```python
from build123d import *

# Parameters (mm, degrees)
SKETCH1_R           = 3.4
SKETCH1_R_2         = 2.45
BOSS_EXTRUDE1_DEPTH = 5.5
BOSS_EXTRUDE2_START = -1.5
SKETCH2_R           = 8.4
SKETCH2_R_2         = 3.4
BOSS_EXTRUDE2_DEPTH = 1.5
FILLET1_R           = 2
FILLET2_R           = 2


with BuildPart() as part:
    # Sketch1 → Boss-Extrude1 (new body)
    with BuildSketch(Plane.XY):
        Circle(SKETCH1_R)
        Circle(SKETCH1_R_2, mode=Mode.SUBTRACT)
    extrude(amount=BOSS_EXTRUDE1_DEPTH)

    # Sketch2 → Boss-Extrude2 (add)
    with BuildSketch(Plane.XY.offset(5.5).offset(BOSS_EXTRUDE2_START)):
        Circle(SKETCH2_R)
        Circle(SKETCH2_R_2, mode=Mode.SUBTRACT)
    extrude(amount=BOSS_EXTRUDE2_DEPTH)

    # Fillet1
    fillet1_edges = [part.edges().sort_by_distance(p)[0] for p in [
        (-3.4, 0, 4),
    ]]
    fillet(fillet1_edges, radius=FILLET1_R)

    # Fillet2
    fillet2_edges = [part.edges().sort_by_distance(p)[0] for p in [
        (-2.45, 0, 5.5),
    ]]
    fillet(fillet2_edges, radius=FILLET2_R)


solid = part.part
```
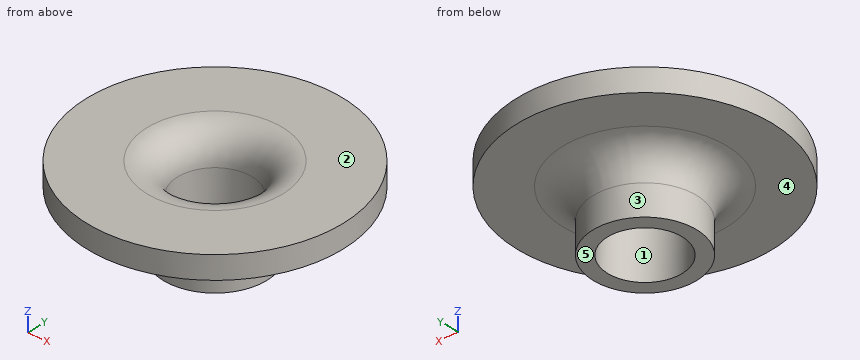
Part model, mm, in its own coordinate system. Face numbers are marked on the shaded views. A direction names the side the tool comes from. Coordinates: 2 decimals unless noted, no trailing zeros. Loops run counter-clockwise (first coordinate to the right, second up) from the corner with the lowest first, then second, coordinate; pieces in that order, holes last. Notation, with made-up numbers: (-39, -0.75) - (-31, -0.75) arc R16 ccw to (-31, 27.25) - close; hole circle Ø4 at (59, -27). An arc over 180 degrees is marked (long way). Write item = value, one per line. Start each with the question number.
Item 1: Cut at A-A, the plane y = 0. Give the cut face in (x, z).
Item 2: 3-axis set-ups, long thin cutter, end or side, ignore diameter. For the marked faces 4 and 5: which of +Z, -Z, +X, -X, +Y, -Y reach the whole face in a straight line?
Item 3: Flat gauge pins, fed straight in: pin 1 Ø2 at (y, z) = (5.5, 4.5) entering from -X; pin 2 Ø1.5 at (y, z) = (6.5, 2) entering from -X; pin 3 Ø1.5 at (x, y) = (3.5, 6.5) entering from -Z. Where does each tip first touch, or does it go through?
Item 4: Mould opens along X. For the marked faces 1, 2 and 3 say: released by +X, released by -X, zero draft, split by the parting line, or undercut.
Item 5: Wall check: L1, parallel to Y at x = 0, z = 1.1; L2, parallel to Z at x = 2.25, y = 6.5; L3, parallel to Y at x = 1.5, z = 0.5. Give the ranges that are in metal, low to high. Write a range as from..to.
Item 6: Cut at C-C, the plane z = 4.7. Give the cut face in (x, y).
Item 7: Cut at D-D, the plane x = 7.25. Give the cut face in (y, z).
The answers:
q1.outline = (-8.4, 4) - (-5.4, 4) arc R2 cw to (-3.4, 2) - (-3.4, 0) - (-2.45, 0) - (-2.45, 3.5) arc R2 ccw to (-4.45, 5.5) - (-8.4, 5.5) - close; (2.45, 0) - (3.4, 0) - (3.4, 2) arc R2 cw to (5.4, 4) - (8.4, 4) - (8.4, 5.5) - (4.45, 5.5) arc R2 ccw to (2.45, 3.5) - close
q2.face_4 = -Z
q2.face_5 = -Z, +X, -X, +Y, -Y
q3.pin_1 = -7.09
q3.pin_2 = through
q3.pin_3 = 4
q4.face_1 = undercut
q4.face_2 = zero draft
q4.face_3 = split by the parting line
q5.L1 = -3.4..-2.45, 2.45..3.4
q5.L2 = 4..5.5
q5.L3 = -3.05..-1.94, 1.94..3.05
q6.outline = circle Ø16.8 at (0, 0); hole circle Ø5.7 at (0, 0)
q7.outline = (-4.24, 4) - (4.24, 4) - (4.24, 5.5) - (-4.24, 5.5) - close
